from build123d import *

# Parameters (mm, degrees)
SKETCH_2_W          = 74
SKETCH_2_H          = 74
EXTRUDE_1_DEPTH     = 2
SKETCH_3_R          = 15
EXTRUDE_2_DEPTH     = 3
SKETCH_4_R          = 12.5
CUT_EXTRUDE_1_DEPTH = 10
M3X0_5_1_D          = 2.5


with BuildPart() as part:
    # ｽｹｯﾁ2 → ﾎﾞｽ - 押し出し1 (new body)
    with BuildSketch(Plane.XY):
        with Locations((-37, -37)):
            Rectangle(SKETCH_2_W, SKETCH_2_H)
    extrude(amount=EXTRUDE_1_DEPTH)

    # ｽｹｯﾁ3 → ﾎﾞｽ - 押し出し2 (add)
    with BuildSketch(Plane.XY.offset(2)):
        with Locations(Location((-37, -37, 0), (0, 0, 180))):
            Circle(SKETCH_3_R)
    extrude(amount=EXTRUDE_2_DEPTH)

    # ｽｹｯﾁ4 → ｶｯﾄ - 押し出し1 (cut)
    with BuildSketch(Plane.XY.offset(5)):
        with Locations((-37, -37)):
            Circle(SKETCH_4_R)
    extrude(amount=-CUT_EXTRUDE_1_DEPTH, mode=Mode.SUBTRACT)

    # M3x0.5 ねじ穴1 (through all)
    with Locations(Plane.XY.offset(2)):
        with Locations((-67, -67), (-7, -67)):
            m3x0_5_1 = Hole(M3X0_5_1_D / 2)

    # ﾐﾗｰ1: M3x0.5 ねじ穴1 across plane
    add(m3x0_5_1.mirror(Plane.ZX.offset(-37)), mode=Mode.SUBTRACT)


solid = part.part
Input: part model. Units: mm. Frame: model coordinates. A direction names the side the tool comes from. Round coordinates to 2 decimals unless told otherwise and drop trailing zeros. Order: outer loops, then holes, each group sorted by start corner. A loop starts at its lowest first (then second) coordinate and runs counter-clockwise, first axis right, second up.
1. Set-up query: faces 5 (the face through (-54, -36, 2)), 6 (the face through (-33.6, -49.3, 5)). Return all of +Z, -Z, +X, -X, +Y, -Y with unobstructed straight access to the full face (end or side cutting, diameter ignored); none if empty.
The answers:
face 5: +Z
face 6: +Z, +X, -X, +Y, -Y
2. Material intervals for line 1 (Y direction, x = -67, z = 0.55); line 2 (Z direction, x = -53.5, y = -6); line 3 (Y direction, x = -30, z = 2.8), sorted ascending.
The answers:
line 1: y = -74 to -68.25, -65.75 to -8.25, -5.75 to 0
line 2: z = 0 to 2
line 3: y = -50.27 to -47.36, -26.64 to -23.73
3. Cut plane B-B, the plane y = -7. Output: boundary loops of the cut face in (x, z), then the cut area to 3 significant figures.
The answers:
outline: (-74, 0) - (-68.25, 0) - (-68.25, 2) - (-74, 2) - close; (-65.75, 0) - (-8.25, 0) - (-8.25, 2) - (-65.75, 2) - close; (-5.75, 0) - (0, 0) - (0, 2) - (-5.75, 2) - close
area: 138 mm2
4. Cut plane A-A, the plane x = -37. Output: boundary loops of the cut face in (y, z), then the cut area to 3 significant figures.
The answers:
outline: (-74, 0) - (-49.5, 0) - (-49.5, 5) - (-52, 5) - (-52, 2) - (-74, 2) - close; (-24.5, 0) - (0, 0) - (0, 2) - (-22, 2) - (-22, 5) - (-24.5, 5) - close
area: 113 mm2
5. Cut plane D-D, the plane z = 0.75. Output: boundary loops of the cut face in (x, y).
The answers:
outline: (-74, -74) - (0, -74) - (0, 0) - (-74, 0) - close; hole circle Ø2.5 at (-67, -67); hole circle Ø2.5 at (-67, -7); hole circle Ø25 at (-37, -37); hole circle Ø2.5 at (-7, -67); hole circle Ø2.5 at (-7, -7)
6. Mould query, pull axis X, two halves, no side actions, for faces 1 (the face through (-25.944, -47.138, 3.479)), 2 (the face through (-68.155, -6.521, 0.986)), 3 (the face through (-74, -38, 1)), 4 (the face through (-54, -36, 0)). Classes: released by +X, released by -X, zero draft, split by the parting line, or undercut.
The answers:
face 1: split by the parting line
face 2: undercut
face 3: released by -X
face 4: zero draft
7. Pin query (flat end, axial travel): P1, Ø1.5, axis at x = -7, y = -7, coming from the -Z side; P2, Ø4, axis at x = -15, y = -26, coming from the +Z side. Return the tip coordinate at first contact, or that it passes through.
The answers:
P1: passes through
P2: stops at z = 2
